Can you work these out from the model? Positions are in its coordinate system, mm. Face numbers are marked on the shaded views. A direction names the side the tool comes from. Round coordinates to 2 decimals unless told otherwise and drop trailing zeros. Loops run counter-clockwise (first coordinate to the right, second up) from the corner with the lowest first, then second, coordinate; pieces in that order, holes last.
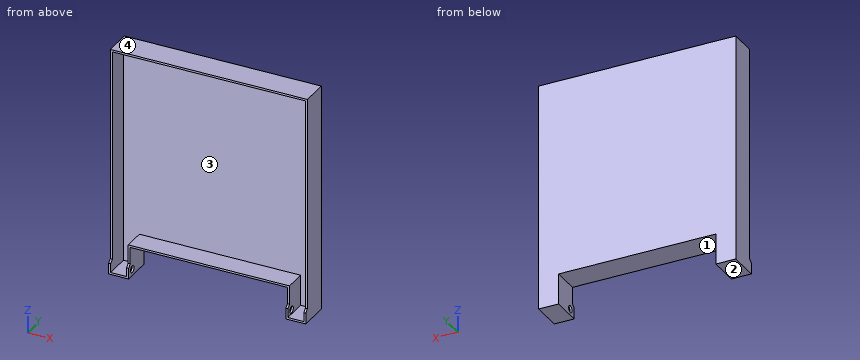
Autodesk Inventor part; units mm, degrees
ref_plane "YZ Plane" through (0, 0, 0) normal (1, 0, 0) x (0, 1, 0)
ref_plane "XZ Plane" through (0, 0, 0) normal (0, 1, 0) x (-1, 0, 0)
ref_plane "XY Plane" through (0, 0, 0) normal (0, 0, 1) x (1, 0, 0)
sketch "Sketch1" plane through (0, 0, 0) normal (0, 1, 0) x (-1, 0, 0)
  line L0 (0, 0) -> (-436, 0)
  line L1 (-436, 0) -> (-436, -437)
  line L2 (-392, -437) -> (-44, -437)
  line L3 (0, -437) -> (0, 0)
  line L4 (0, -437) -> (0, -505)
  line L5 (0, -505) -> (-44, -505)
  line L6 (-44, -505) -> (-44, -437)
  line L7 (-436, -437) -> (-436, -505)
  line L8 (-436, -505) -> (-392, -505)
  line L9 (-392, -505) -> (-392, -437)
  dimension "d0" = 436
  dimension "d1" = 437
  dimension "d2" = 68
  dimension "d3" = 44
  dimension "d4" = 68
  dimension "d5" = 68
  dimension "d6" = 44
  dimension "d7" = 68
extrude "Extrusion1" add sketch "Sketch1" along normal blind 67
sketch "Sketch4" plane through (436, 0, 0) normal (1, 0, 0) x (0, 0, -1)
  line L0 (504.9333, 0) -> (480.9333, 0)
  line L1 (505, 0) -> (437, 0)
  line L2 (480.9333, 0) -> (473.8622, 7.0711)
  line L3 (473.8622, 7.0711) -> (0, 7.0711)
  line L4 (0, 0) -> (0, 67)
  line L5 (0, 7.0711) -> (0, 0)
  line L6 (0, 0) -> (480.9333, 0)
  dimension "d13" = 24
  dimension "d14" = 10
  dimension "d15" = 135
extrude "Extrusion2" cut sketch "Sketch4" against normal through all
sketch "Sketch5" plane through (0, 0, 0) normal (0, -1, 0) x (1, 0, 0)
  line L0 (0, 0) -> (436, 0)
  line L1 (436, 0) -> (0, 0)
  line L2 (0, -505) -> (0, -480.9333)
  line L3 (0, 0) -> (0, -505)
  line L4 (44, -505) -> (0, -505)
  line L5 (0, -505) -> (44, -505)
  line L6 (44, -437) -> (44, -505)
  line L7 (44, -505) -> (44, -437)
  line L8 (392, -505) -> (392, -437)
  line L9 (44, -437) -> (392, -437)
  line L10 (392, -437) -> (392, -505)
  line L11 (436, -505) -> (392, -505)
  line L12 (392, -505) -> (436, -505)
  line L13 (436, 0) -> (436, -505)
  line L14 (436, -505) -> (436, 0)
  line L15 (396.4, -432.6) -> (39.6, -432.6)
  line L16 (39.6, -432.6) -> (39.6, -500.6)
  line L17 (39.6, -500.6) -> (4.4, -500.6)
  line L18 (4.4, -500.6) -> (4.4, -4.4)
  line L19 (4.4, -4.4) -> (431.6, -4.4)
  line L20 (431.6, -4.4) -> (431.6, -500.6)
  line L21 (431.6, -500.6) -> (396.4, -500.6)
  line L22 (396.4, -500.6) -> (396.4, -432.6)
  dimension "d18" = 4.4
extrude "Extrusion3" cut sketch "Sketch5" against normal blind 55 contours L15 L16 L17 L18 L19 L20 L21 L22
sketch "Sketch3" plane through (44, 0, -437) normal (1, 0, 0) x (0, 0, -1)
  circle A0 centre (54, 16) radius 7.5
  line L0 (0, 0) -> (0, 67)
  line L1 (0, 0) -> (68, 0)
  point P0 (-437, 0)
  dimension "d10" = 15
  dimension "d11" = 54
  dimension "d12" = 16
extrude "Extrusion4" cut sketch "Sketch3" along normal blind 367.5 and the other way blind 27.5
properties part number "bin_lid"
(1) If we mould it in two halves opening along X, with no side actions, what happens to the marked faces 3 and 4? For each: released by +X, released by -X, zero draft, split by the parting line, or undercut.
Worked answers:
face 3: undercut
face 4: zero draft
(2) If we section it at A-A, the plane z = -491: List the corners of the cut face in (x, y) for me.
Worked answers:
outline: (0, 0) - (4.4, 0) - (4.4, 55) - (39.6, 55) - (39.6, 23.5) - (44, 23.5) - (44, 67) - (0, 67) - close; (39.6, 0) - (44, 0) - (44, 8.5) - (39.6, 8.5) - close; (392, 0) - (396.4, 0) - (396.4, 8.5) - (392, 8.5) - close; (392, 23.5) - (396.4, 23.5) - (396.4, 55) - (431.6, 55) - (431.6, 0) - (436, 0) - (436, 67) - (392, 67) - close
(3) Will these pins go through, and if not, where does the flat tip stop? P1, Ø5, axis at x = 183, y = 37.5, coming from the +Z side; P2, Ø10, axis at x = 79.5, y = 16.5, coming from the -Z side; P3, Ø3, axis at x = 257, z = -324.5, coming from the -Y side.
Worked answers:
P1: stops at z = 0
P2: stops at z = -437
P3: stops at y = 55
(4) If we section it at B-B, the plane y = 16: List the corners of the cut face in (x, z) for me.
Worked answers:
outline: (0, -505) - (44, -505) - (44, -498.5) - (39.6, -498.5) - (39.6, -500.6) - (4.4, -500.6) - (4.4, -4.4) - (431.6, -4.4) - (431.6, -500.6) - (396.4, -500.6) - (396.4, -498.5) - (392, -498.5) - (392, -505) - (436, -505) - (436, 0) - (0, 0) - close; (39.6, -483.5) - (44, -483.5) - (44, -437) - (392, -437) - (392, -483.5) - (396.4, -483.5) - (396.4, -432.6) - (39.6, -432.6) - close
(5) For the marked faces 1 and 2, which set-ups out of +Z, -Z, +X, -X, +Y, -Y let a thin tool reach every point of the face, with its end or its side?
Worked answers:
face 1: -Z, +Y, -Y
face 2: -Z, +X, -X, +Y, -Y
(6) If we section it at C-C, the plane x = 65: List the corners of the cut face in (y, z) for me.
Worked answers:
outline: (7.07, -437) - (67, -437) - (67, 0) - (7.07, 0) - (7.07, -4.4) - (55, -4.4) - (55, -432.6) - (7.07, -432.6) - close
(7) If we section it at D-D, the plane z = -421: List the corners of the cut face in (x, y) for me.
Worked answers:
outline: (0, 7.07) - (4.4, 7.07) - (4.4, 55) - (431.6, 55) - (431.6, 7.07) - (436, 7.07) - (436, 67) - (0, 67) - close
(8) If I drill on line 1 (Z direction, x = 393.45, y = 16); line 2 (X direction, y = 22, z = -463.5); line 3 (Z direction, x = 407, y = 14), over which ranges is the centre line in solid material (lowest first)?
Worked answers:
line 1: z = -505 to -498.5, -483.5 to -432.6, -4.4 to 0
line 2: x = 0 to 4.4, 39.6 to 44, 392 to 396.4, 431.6 to 436
line 3: z = -505 to -500.6, -4.4 to 0
